from build123d import *

# Parameters (mm, degrees)
SKETCH1_W           = 23
SKETCH1_H           = 12
BOSS_EXTRUDE1_DEPTH = 22.5
SKETCH2_W           = 12
SKETCH2_H           = 2.5
BOSS_EXTRUDE2_DEPTH = 5
CUT_EXTRUDE1_DEPTH  = 5
BOSS_EXTRUDE3_DEPTH = 6
FILLET1_R           = 5
SKETCH5_R           = 1.75
BOSS_EXTRUDE4_DEPTH = 4
SKETCH6_R           = 1.25
CUT_EXTRUDE2_DEPTH  = 4


with BuildPart() as part:
    # Sketch1 → Boss-Extrude1 (new body)
    with BuildSketch(Plane(origin=(0, 0, 0), x_dir=(1, 0, 0), z_dir=(0, 1, 0))):
        Rectangle(SKETCH1_W, SKETCH1_H)
    extrude(amount=BOSS_EXTRUDE1_DEPTH)

    # Sketch2 → Boss-Extrude2 (add)
    with BuildSketch(Plane(origin=(11.5, 0, 0), x_dir=(0, 0, -1), z_dir=(1, 0, 0))):
        with Locations((0, 19.25)):
            Rectangle(SKETCH2_W, SKETCH2_H)
    boss_extrude2 = extrude(amount=BOSS_EXTRUDE2_DEPTH)

    # Sketch3 → Cut-Extrude1 (cut)
    with BuildSketch(Plane(origin=(0, 20.5, 0), x_dir=(1, 0, 0), z_dir=(0, 1, 0))):
        with BuildLine():
            Line((15.645643924, 0.5), (16.5, 0.5))
            Line((16.5, 0.5), (16.5, -0.5))
            Line((16.5, -0.5), (15.645643924, -0.5))
            ThreePointArc((15.645643924, -0.5), (13.25, 0), (15.645643924, 0.5))
        make_face()
    cut_extrude1 = extrude(amount=-CUT_EXTRUDE1_DEPTH, mode=Mode.SUBTRACT)

    # Mirror1: Boss-Extrude2, Cut-Extrude1 across plane
    add(boss_extrude2.mirror(Plane(origin=(0, 0, 0), x_dir=(0, 0, 1), z_dir=(1, 0, 0))))
    add(cut_extrude1.mirror(Plane(origin=(0, 0, 0), x_dir=(0, 0, 1), z_dir=(1, 0, 0))), mode=Mode.SUBTRACT)

    # Sketch4 → Boss-Extrude3 (add)
    with BuildSketch(Plane(origin=(0, 22.5, 0), x_dir=(1, 0, 0), z_dir=(0, 1, 0))):
        with BuildLine():
            Line((-8.5, 6), (4.5, 6))
            Line((4.5, 6), (4.5, -6))
            Line((4.5, -6), (-8.5, -6))
            ThreePointArc((-8.5, -6), (-10.621320344, -5.121320344), (-11.5, -3))
            Line((-11.5, -3), (-11.5, 3))
            ThreePointArc((-11.5, 3), (-10.621320344, 5.121320344), (-8.5, 6))
        make_face()
    extrude(amount=BOSS_EXTRUDE3_DEPTH)

    # Fillet1
    fillet1_edges = [part.edges().sort_by_distance(p)[0] for p in [
        (4.5, 25.5, 6),
        (4.5, 25.5, -6),
    ]]
    fillet(fillet1_edges, radius=FILLET1_R)

    # Sketch5 → Boss-Extrude4 (add)
    with BuildSketch(Plane(origin=(0, 28.5, 0), x_dir=(1, 0, 0), z_dir=(0, 1, 0))):
        with Locations(Location((-5, 0, 0), (0, 0, 270))):
            Circle(SKETCH5_R)
    extrude(amount=BOSS_EXTRUDE4_DEPTH)

    # Sketch6 → Cut-Extrude2 (cut)
    with BuildSketch(Plane(origin=(0, 32.5, 0), x_dir=(1, 0, 0), z_dir=(0, 1, 0))):
        with Locations(Location((-5, 0, 0), (0, 0, 270))):
            Circle(SKETCH6_R)
    extrude(amount=-CUT_EXTRUDE2_DEPTH, mode=Mode.SUBTRACT)


solid = part.part
Verification items for the finished model (mm, model axes). A direction names the side the tool comes from. Coordinates: 2 decimals unless noted, no trailing zeros. Order: outer loops, then holes, each group sorted by start corner. A loop starts at its lowest first (then second) coordinate and runs counter-clockwise, first axis right, second up. Notation, with made-up numbers: M 80,-11.5 L 131,-11.5 A28 ccw 131,20.5 Z; hole C 64,35.25 d11. An arc over 180 degrees is marked long. One line per item, written item: value. Start each with the question number.
Item 1: Sectioned sample at A-A (x = 14.5). Enter the section's corners in (y, z).
Item 2: Mould release check, pull along X, two halves, no side actions. Record for faces 6 (the cylindrical face through (13.25, 19.27, 0.05)), 7 (the flat face through (-16.5, 19, -3)), 8 (the cylindrical face through (3, 25.54, -4.57)), 9 (the cylindrical face through (-6.22, 30.53, -0.27)): released by +X, released by -X, zero draft, split by the parting line, or undercut.
Item 3: Sectioned sample at C-C (z = 0). Enter the section's corners in (x, y).
Item 4: Gauge pin test, flat ends, axial feed: pin 1 (2.5 mm diameter, centred on x = -10, z = -5, fed in from +Y); pin 2 (4 mm diameter, centred on x = 14.5, z = 0, fed in from -Y); pin 3 (6.5 mm diameter, centred on y = 26, z = 0, fed in from -X). Record the tip position at first contact, or that the pin passes through.
Item 5: Access from +Z, -Z, +X, -X, +Y, -Y to the whole of each face (thin tool, end or side, straight path). Record for faces 1 (the cylindrical face through (3, 25.54, 4.57)), 2 (the flat face through (-16, 19, -0.5)), 3 (the flat face through (-13, 20.5, 0)), 4 (the flat face through (11.5, 21, 0)), 5 (the flat face through (-13, 18, 0)).
Item 6: Sectioned sample at D-D (x = -5). Enter the section's corners in (y, z), then the cut area to 3 significant figures.
Item 7: Sectioned sample at B-B (y = 26.5). Enter the section's corners in (x, z).
Item 8: Scan lines: probe 1 along X at (y, z) = (29.4, 0); probe 2 along Z at (x, y) = (14.5, 19.05); probe 3 along Y at (x, z) = (-10, -5). Record each from-to range of solid material in increasing order.
Conclusion:
1. outline: M 18,-6 L 20.5,-6 L 20.5,-1.25 L 18,-1.25 Z; M 18,1.25 L 20.5,1.25 L 20.5,6 L 18,6 Z
2. face 6: undercut
2. face 7: released by -X
2. face 8: released by +X
2. face 9: undercut
3. outline: M -13.25,18 L -11.5,18 L -11.5,0 L 11.5,0 L 11.5,18 L 13.25,18 L 13.25,20.5 L 11.5,20.5 L 11.5,22.5 L 4.5,22.5 L 4.5,28.5 L -3.25,28.5 L -3.25,32.5 L -3.75,32.5 L -3.75,28.5 L -6.25,28.5 L -6.25,32.5 L -6.75,32.5 L -6.75,28.5 L -11.5,28.5 L -11.5,20.5 L -13.25,20.5 Z
4. pin 1: stops at y = 28.5
4. pin 2: stops at y = 18
4. pin 3: stops at x = -11.5
5. face 1: +Z, +X, +Y
5. face 2: -X, +Y, -Y
5. face 3: +Z, -Z, -X, +Y
5. face 4: +Z, -Z, +X, +Y
5. face 5: +Z, -Z, -X, -Y
6. outline: M 0,-6 L 28.5,-6 L 28.5,-1.75 L 32.5,-1.75 L 32.5,-1.25 L 28.5,-1.25 L 28.5,1.25 L 32.5,1.25 L 32.5,1.75 L 28.5,1.75 L 28.5,6 L 0,6 Z
6. area: 346 mm^2
7. outline: M -11.5,-3 A3 ccw -8.5,-6 L -0.5,-6 A5 ccw 4.5,-1 L 4.5,1 A5 ccw -0.5,6 L -8.5,6 A3 ccw -11.5,3 Z
8. probe 1: x = -6.75 to -6.25, -3.75 to -3.25
8. probe 2: z = -6 to -1.25, 1.25 to 6
8. probe 3: y = 0 to 28.5
